Design review of the part built by this model. Coordinates are the model's own, in mm. Face numbers are marked on the shaded views. A direction names the side the tool comes from. Coordinates: 2 decimals unless noted, no trailing zeros. Loops run counter-clockwise (first coordinate to the right, second up) from the corner with the lowest first, then second, coordinate; pieces in that order, holes last.
Q1. For P1, Ø3, axis at x = 8.5, z = 19, coming from the +Y side (3 decimals); P2, Ø1, axis at y = -46.5, z = 0.5, coming from the -X side; P3, Ø8, axis at x = 13, z = 12, coming from the -Y side, all flat-tipped, find the tip position at first contact; note any pin that passes through.
Q2. Add section A-A on x = 24.5. Give the boundary of the cut face in (y, z) (3 decimals).
Q3. Machinability: for the marked faces 4, 5 and 6, which of the approach directions +Z, -Z, +X, -X, +Y, -Y give a long, thin tool a straight path to every point of the face, cutting with its end or side? Answer none if there is none.
Q4. Wall thickness on probe 1 along Y at (x, z) = (-25, 52) (3 decimals); probe 2 along Z at (x, y) = (64, 0); probe 3 along X at (y, z) = (65, -7): over which ranges is each line inside the solid? List them lowest first.
Q5. Add section B-B on z = 0. Give the boundary of the cut face in (x, y) (3 decimals), and give its area (3 significant figures).
Q6. Draft analysis for pull direction Z (two halves, no side actions). For the marked faces 1, 2 and 3, state which applies: released by +Z, released by -Z, zero draft, split by the parting line, or undercut.
Q7. Add section D-D on x = 0. Give the boundary of the cut face in (y, z) (3 decimals), and give its area (3 significant figures).
Q8. Add section C-C on y = 0. Give the boundary of the cut face in (x, z), and give its area (3 significant figures).
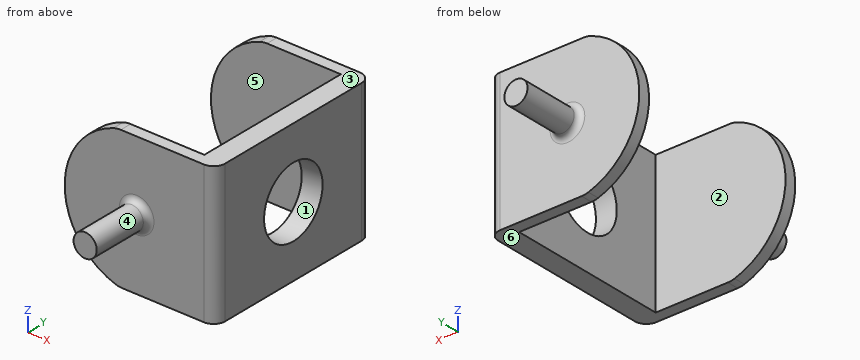
```python
from build123d import *

# Parameters (mm, degrees)
SWEEP1_PROFILE_R    = 10
SKETCH8_R           = 10
BOSS_EXTRUDE1_DEPTH = 0.25
BOSS_EXTRUDE2_DEPTH = 10
BOSS_EXTRUDE5_DEPTH = 120
SKETCH15_W          = 120
SKETCH15_H          = 140
CUT_EXTRUDE2_DEPTH  = 95
FILLET1_R           = 5
FILLET3_R           = 20
FILLET4_R           = 10
SKETCH16_R          = 30
CUT_EXTRUDE3_DEPTH  = 18


with BuildPart() as part:
    # Sweep1: sweep along a path in Sketch1
    with BuildLine(Plane.XY) as sweep1_path:
        Line((0, 132.640900072), (0, -132.640900072))
    # Sweep1 profile (on start of the path) → Sweep1 (sweep)
    with BuildSketch(Plane(origin=(0, 132.640900072, 0), x_dir=(-1, 0, 0), z_dir=(0, -1, 0))):
        Circle(SWEEP1_PROFILE_R)
    sweep(path=sweep1_path.line)

    # Sketch8 → Boss-Extrude1 (add)
    with BuildSketch(Plane(origin=(0, 132.640900072, 0), x_dir=(1, 0, 0), z_dir=(0, 1, 0))):
        Circle(SKETCH8_R)
    extrude(amount=BOSS_EXTRUDE1_DEPTH)

    # Sketch9 → Boss-Extrude2 (add)
    with BuildSketch(Plane(origin=(0, 80.125, 0), x_dir=(1, 0, 0), z_dir=(0, 1, 0))):
        with BuildLine():
            Line((60, -59.786486662), (-16.583123952, -59.786486662))
            ThreePointArc((-16.583123952, -59.786486662), (-62.038041158, 0.839902741), (-14.958502558, 60.213513338))
            Line((-14.958502558, 60.213513338), (60, 60.213513338))
            Line((60, 60.213513338), (60, -59.786486662))
        make_face()
    boss_extrude2 = extrude(amount=-BOSS_EXTRUDE2_DEPTH)

    # Mirror1: Boss-Extrude2 across plane
    add(boss_extrude2.mirror(Plane.ZX.offset(0.125)))

    # Sketch14 → Boss-Extrude5 (add)
    with BuildSketch(Plane.XY.offset(59.786486662)):
        Polygon((50, 70.125), (60, 70.125), (60, 80.125), (68, 80.125), (68, -79.875), (60, -79.875), (60, -69.875), (50, -69.875), align=None)
    extrude(amount=-BOSS_EXTRUDE5_DEPTH)

    # Sketch15 → Cut-Extrude2 (cut)
    with BuildSketch(Plane.ZY.offset(-50)):
        with Locations((-0.213513338, 0.125)):
            Rectangle(SKETCH15_W, SKETCH15_H)
    extrude(amount=CUT_EXTRUDE2_DEPTH, mode=Mode.SUBTRACT)

    # Fillet1
    fillet1_edges = [part.edges().sort_by_distance(p)[0] for p in [
        (10, 80.125, 0),
        (10, -79.875, 0),
    ]]
    fillet(fillet1_edges, radius=FILLET1_R)

    # Fillet3
    fillet3_edges = [part.edges().sort_by_distance(p)[0] for p in [
        (-16.583123952, 75.125, 59.786486662),
        (-14.958502558, 75.125, -60.213513338),
        (-14.958502558, -74.875, -60.213513338),
        (-16.583123952, -74.875, 59.786486662),
    ]]
    fillet(fillet3_edges, radius=FILLET3_R)

    # Fillet4
    fillet4_edges = [part.edges().sort_by_distance(p)[0] for p in [
        (68, 80.125, -0.213513338),
        (68, -79.875, -0.213513338),
    ]]
    fillet(fillet4_edges, radius=FILLET4_R)

    # Sketch16 → Cut-Extrude3 (cut)
    with BuildSketch(Plane(origin=(68, 0, 0), x_dir=(0, 0, -1), z_dir=(1, 0, 0))):
        with Locations(Location((0, 0, 0), (0, 0, 90))):
            Circle(SKETCH16_R)
    extrude(amount=-CUT_EXTRUDE3_DEPTH, mode=Mode.SUBTRACT)


solid = part.part
```
Entries:
1. P1: stops at y = 80.125
1. P2: stops at x = 50
1. P3: stops at y = -80.05
2. outline: (-79.875, -60.214) - (-69.875, -60.214) - (-69.875, 59.786) - (-79.875, 59.786) - close; (70.125, -60.214) - (80.125, -60.214) - (80.125, 59.786) - (70.125, 59.786) - close
3. face 4: -Y
3. face 5: +Z, -Z, -X
3. face 6: -Z, +X, -X, +Y, -Y
4. probe 1: y = -79.875 to -69.875, 70.125 to 80.125
4. probe 2: z = -60.21 to -30, 30 to 59.79
4. probe 3: x = 50 to 68
5. outline: (-62.044, -79.875) - (-15, -79.875) arc R5 cw to (-10, -84.875) - (-10, -132.641) - (10, -132.641) - (10, -84.875) arc R5 cw to (15, -79.875) - (58, -79.875) arc R10 ccw to (68, -69.875) - (68, -30) - (50, -30) - (50, -69.875) - (-62.044, -69.875) - close; (-62.044, 70.125) - (50, 70.125) - (50, 30) - (68, 30) - (68, 70.125) arc R10 ccw to (58, 80.125) - (15, 80.125) arc R5 cw to (10, 85.125) - (10, 132.891) - (-10, 132.891) - (-10, 85.125) arc R5 cw to (-15, 80.125) - (-62.044, 80.125) - close
5. area: 6,130 mm2
6. face 1: undercut
6. face 2: zero draft
6. face 3: released by +Z
7. outline: (-132.641, -10) - (-84.875, -10) arc R5 cw to (-79.875, -15) - (-79.875, -60.214) - (-69.875, -60.214) - (-69.875, 59.786) - (-79.875, 59.786) - (-79.875, 15) arc R5 cw to (-84.875, 10) - (-132.641, 10) - close; (70.125, -60.214) - (80.125, -60.214) - (80.125, -15) arc R5 cw to (85.125, -10) - (132.891, -10) - (132.891, 10) - (85.125, 10) arc R5 cw to (80.125, 15) - (80.125, 59.786) - (70.125, 59.786) - close
7. area: 4,530 mm2
8. outline: (50, -60.21) - (68, -60.21) - (68, -30) - (50, -30) - close; (50, 30) - (68, 30) - (68, 59.79) - (50, 59.79) - close
8. area: 1,080 mm2
